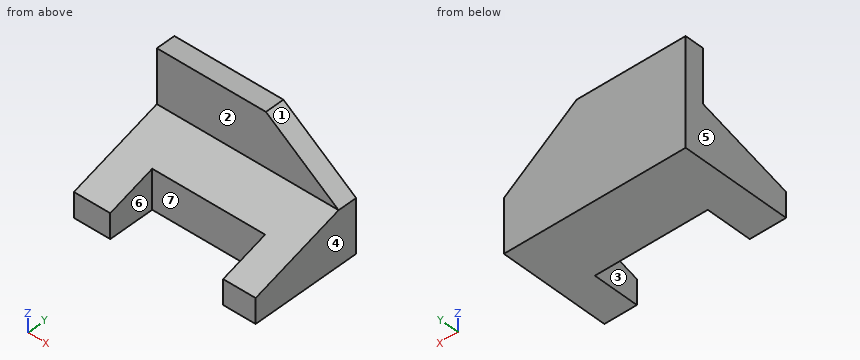
from build123d import *

# Parameters (mm, degrees)
F0_W     = 10
F0_H     = 28
F1_DEPTH = 95
F3_DEPTH = 10
F4_W     = 59
F4_H     = 24
F5_DEPTH = 62.4


with BuildPart() as f1:
    # F0 (on Right) → F1 (new body)
    with BuildSketch(Plane.YZ):
        Polygon((-57.430514, 0), (0, 0), (0, 28), (-10, 28), (-57.430514, 13), align=None)
        with Locations((-5, 42)):
            Rectangle(F0_W, F0_H)
    extrude(amount=-F1_DEPTH)

    # F2 (on face) → F3 (cut)
    with BuildSketch(Plane.XZ.offset(10)):
        Polygon((0, 56), (-37.998203, 56), (0, 28), align=None)
    extrude(amount=-F3_DEPTH, mode=Mode.SUBTRACT)

    # F4 (on face) → F5 (cut)
    with BuildSketch(Plane(origin=(0, 0, 0), x_dir=(1, 0, 0), z_dir=(0, 0, -1))):
        with Locations((-46.5, 45.430514)):
            Rectangle(F4_W, F4_H)
    extrude(amount=-F5_DEPTH, mode=Mode.SUBTRACT)


solid = f1.part
Verification items for the finished model (mm, model axes). Face numbers are marked on the shaded views. A direction names the side the tool comes from. Give positions to 0.01 mm unless a question says otherwise; leave off trailing zeros. Order: outer loops, then holes, each group sorted by start corner. A loop starts at its lowest first (then second) coordinate and runs counter-clockwise, first axis right, second up. Notation, with made-up numbers: M 25,-2 L 79,-2 A11 cw 79,2 Z; hole C 32.5,13 d1. An arc over 180 degrees is marked long. Answer as a JSON object with one key per item and string values. Group by question number.
1) Depth check by flat-ended pin: pin 1 Ø12 at (x, y) = (-14.5, -24) entering from +Z; pin 2 Ø22.5 at (x, z) = (-54, 7) entering from -Y; pin 3 Ø14 at (x, z) = (-26, 40) entering from -Y. Enter the tip coordinate at first touch or a pass-through.
2) Cross-section at A-A (y = -39). Enter the section's corners in (x, z).
3) Mould release check, pull along X, two halves, no side actions. Record for the marked faces 4, 5, 6 and 7: released by +X, released by -X, zero draft, split by the parting line, or undercut.
4) Scan lines: line 1 along X through (y, z) = (-50, 12); line 2 along Y through (x, z) = (-46, 44.5); line 3 along Y through (x, z) = (-40.5, 16.5). Record each from-to range of solid material in increasing order. Write a range as [from, to].
5) Cross-section at D-D (y = -9). Enter the section's corners in (x, z), then the cut area to 3 significant figures.
6) Cross-section at C-C (x = -80.5). Enter the section's corners in (y, z).
7) Cross-section at B-B (z = 9). Enter the section's corners in (x, y).
8) Access from +Z, -Z, +X, -X, +Y, -Y to the whole of each face (thin tool, end or side, straight path). Record for the marked faces 1, 2 and 3.
Result sheet:
{
 "1": {"pin 1": "stops at z = 25.47", "pin 2": "stops at y = -33.43", "pin 3": "stops at y = -10"},
 "2": {"outline": "M -95,0 L -76,0 L -76,18.83 L -95,18.83 Z; M -17,0 L 0,0 L 0,18.83 L -17,18.83 Z"},
 "3": {"face 4": "released by +X", "face 5": "released by -X", "face 6": "undercut", "face 7": "undercut"},
 "4": {"line 1": "x = [-95, -76], [-17, 0]", "line 2": "y = [-10, 0]", "line 3": "y = [-33.43, 0]"},
 "5": {"outline": "M -95,0 L 0,0 L 0,28 L -38,56 L -95,56 Z", "area": "4,790 mm2"},
 "6": {"outline": "M -57.43,0 L 0,0 L 0,56 L -10,56 L -10,28 L -57.43,13 Z"},
 "7": {"outline": "M -95,-57.43 L -76,-57.43 L -76,-33.43 L -17,-33.43 L -17,-57.43 L 0,-57.43 L 0,0 L -95,0 Z"},
 "8": {"face 1": "+Z, +X, +Y, -Y", "face 2": "+Z, +X, -X, -Y", "face 3": "+Z, -Z, -Y"}
}
